The drawing under review shows one solid part. Ordinate dimensions are in mm from its lowest x, y, z. Round coordinates to 2 decimals unless told otherwise and drop trailing zeros. Loops run counter-clockwise (first coordinate to the right, second up) from the corner with the lowest first, then second, coordinate; pieces in that order, holes last. Notation, with made-up numbers: M 67,39.5 L 125,39.5 A25 cw 125,61.5 Z; hole C 81.5,81 d11. An arc over 180 degrees is marked long. Use a Markdown table: item, result.
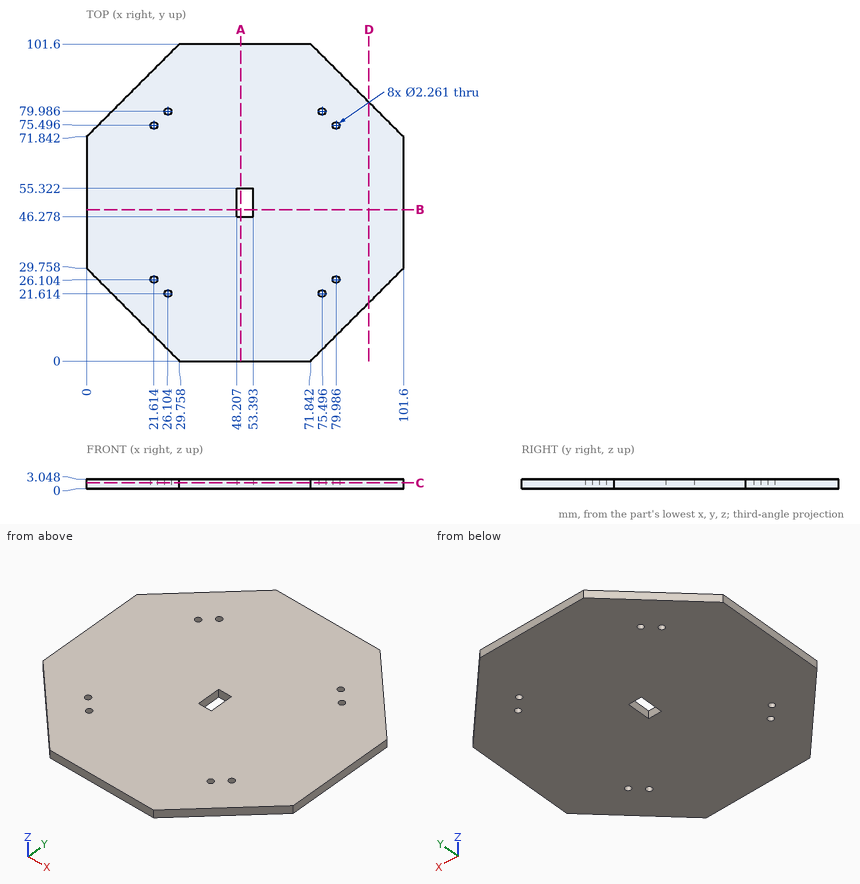
1. Insertion check: pin 1 (1.4 mm diameter, centred on x = 21.61, y = 75.5, fed in from -Z); pin 2 (3 mm diameter, centred on x = 75.5, y = 21.61, fed in from +Z). Each pin has a flat end and moves straight along its axis. Give the tip position at first contact, or say it passes through.
Check values:
| item | result |
|---|---|
| pin 1 | passes through |
| pin 2 | stops at z = 3.05 |
2. Take a section at A-A on x = 49.5. Give the boundary of the cut face in (y, z).
Check values:
| item | result |
|---|---|
| outline | M 0,0 L 46.28,0 L 46.28,3.05 L 0,3.05 Z; M 55.32,0 L 101.6,0 L 101.6,3.05 L 55.32,3.05 Z |
3. Take a section at C-C on z = 1.8. Count the separate pieces of the cut face and the enclosed holes in it, and give its area (3 significant figures).
Check values:
| item | result |
|---|---|
| separate pieces | 1 |
| enclosed holes | 9 |
| area | 8,470 mm² |
4. Take a section at D-D on x = 90.5. Give the boundary of the cut face in (y, z), and give its area (3 significant figures).
Check values:
| item | result |
|---|---|
| outline | M 18.66,0 L 82.94,0 L 82.94,3.05 L 18.66,3.05 Z |
| area | 196 mm² |
5. Wall thickness on line 1 along X through (y, z) = (53.5, 2.75); line 2 along X through (y, z) = (81, 0.3) (1 decimal); line 3 along Y through (x, z) = (82, 1.75): over which ranges is each line inside the solid? List them lowest first. Write a range as from..to.
Check values:
| item | result |
|---|---|
| line 1 | x = 0..48.21, 53.39..101.6 |
| line 2 | x = 9.2..25.6, 26.6..75, 76..92.4 |
| line 3 | y = 10.16..91.44 |
6. Take a section at B-B on y = 48.5. Give the boundary of the cut face in (x, z).
Check values:
| item | result |
|---|---|
| outline | M 0,0 L 48.21,0 L 48.21,3.05 L 0,3.05 Z; M 53.39,0 L 101.6,0 L 101.6,3.05 L 53.39,3.05 Z |
